Can you work these out from the model? Positions are in its coordinate system, mm. A direction names the side the tool comes from. Coordinates: 2 decimals unless noted, no trailing zeros. Order: outer loops, then holes, each group sorted by start corner. A loop starts at its lowest first (then second) coordinate and runs counter-clockwise, first axis right, second up. Notation, with made-up numbers: (-34.5, 41) -> (-25.5, 41) arc R15 cw to (-25.5, 53) -> close; hole circle Ø6 at (7, -5). An arc over 180 degrees is marked (long way). Write item = value, one per line.
```python
from build123d import *

# Parameters (mm, degrees)
SKETCH1_R           = 31.35
SKETCH1_R_2         = 16.65
BOSS_EXTRUDE1_DEPTH = 3
SKETCH2_R           = 4.85
BOSS_EXTRUDE2_DEPTH = 18
CIRPATTERN1_COUNT   = 6
CHAMFER1_SIZE       = 0.6


with BuildPart() as part:
    # Sketch1 → Boss-Extrude1 (new body)
    with BuildSketch(Plane.XY):
        Circle(SKETCH1_R)
        Circle(SKETCH1_R_2, mode=Mode.SUBTRACT)
    extrude(amount=-BOSS_EXTRUDE1_DEPTH)

    # Sketch2 → Boss-Extrude2 (add)
    with BuildSketch(Plane.XY):
        with Locations((24, 0)):
            Circle(SKETCH2_R)
    boss_extrude2 = extrude(amount=BOSS_EXTRUDE2_DEPTH)

    # CirPattern1: Boss-Extrude2 ×6 about axis
    cirpattern1_axis = Axis((0, 0, 0), (0, 0, 1))
    for i in range(1, CIRPATTERN1_COUNT):
        add(boss_extrude2.rotate(cirpattern1_axis, i * 360 / CIRPATTERN1_COUNT))

    # Chamfer1
    chamfer1_edges = [part.edges().sort_by_distance(p)[0] for p in [
        (19.15, 0, 18),
        (9.575, -16.584386482, 18),
        (-9.575, -16.584386482, 18),
        (-31.35, 0, 0),
        (-19.15, 0, 18),
        (-9.575, 16.584386482, 18),
        (9.575, 16.584386482, 18),
        (-31.35, 0, -3),
        (-16.65, 0, -3),
        (-16.65, 0, 0),
    ]]
    chamfer(chamfer1_edges, length=CHAMFER1_SIZE)


solid = part.part
```
Item 1: I want a section at B-B, the plane y = 0. Please give me the cut outline in (x, z), plus the area to 3 significant figures.
A:
outline = (-31.35, -2.4) -> (-30.75, -3) -> (-17.25, -3) -> (-16.65, -2.4) -> (-16.65, -0.6) -> (-17.25, 0) -> (-19.15, 0) -> (-19.15, 17.4) -> (-19.75, 18) -> (-28.25, 18) -> (-28.85, 17.4) -> (-28.85, 0) -> (-30.75, 0) -> (-31.35, -0.6) -> close; (16.65, -2.4) -> (17.25, -3) -> (30.75, -3) -> (31.35, -2.4) -> (31.35, -0.6) -> (30.75, 0) -> (28.85, 0) -> (28.85, 17.4) -> (28.25, 18) -> (19.75, 18) -> (19.15, 17.4) -> (19.15, 0) -> (17.25, 0) -> (16.65, -0.6) -> close
area = 435 mm2
Item 2: I want a section at C-C, the plane z = 12. Please give me the cut outline in (x, y) (3 decimals).
A:
outline = circle Ø9.7 at (-24, 0); circle Ø9.7 at (-12, -20.785); circle Ø9.7 at (-12, 20.785); circle Ø9.7 at (12, -20.785); circle Ø9.7 at (12, 20.785); circle Ø9.7 at (24, 0)
Item 3: If we mould it in two halves opening along Y, with no side actions, what happens to faces 3 (the cylindrical face through (-7.52, 18.93, 8.58)), 4 (the cylindrical face through (7.52, -18.93, 8.58)), 5 (the cylindrical face through (-19.155, -0.213, 8.578)), 6 (the flat face through (-12, 21, 18))? For each: pulls with the +Y half, pulls with the -Y half, needs draft (parallel to the pull), parting line crosses it, or undercut.
A:
face_3 = undercut
face_4 = undercut
face_5 = parting line crosses it
face_6 = needs draft
Item 4: I'm going to push flat-ended pins straight in: P1, Ø1, axis at x = 7.5, y = 16.5, coming from the +Z side; P2, Ø10, axis at x = 9, z = 2, coming from the +Y side; P3, Ø6, axis at x = 11, z = 13, coming from the -Y side; P4, Ø18.5, axis at x = 5.5, y = 4.5, coming from the +Z side. Where does each tip first touch, or does it pass through?
A:
P1 = 0
P2 = 30.99
P3 = -25.63
P4 = through
Item 5: I want a section at A-A, the plane x = 0. Please give me the cut outline in (y, z), plus the area to 3 significant figures.
A:
outline = (-31.35, -2.4) -> (-30.75, -3) -> (-17.25, -3) -> (-16.65, -2.4) -> (-16.65, -0.6) -> (-17.25, 0) -> (-30.75, 0) -> (-31.35, -0.6) -> close; (16.65, -2.4) -> (17.25, -3) -> (30.75, -3) -> (31.35, -2.4) -> (31.35, -0.6) -> (30.75, 0) -> (17.25, 0) -> (16.65, -0.6) -> close
area = 86.8 mm2
Item 6: If I drill on probe 1 along Y at (x, z) = (0, -1.9); probe 2 along Z at (x, y) = (23, 17.5); probe 3 along Y at (x, z) = (13.5, 16.25), over which ranges is the centre line in solid material (lowest first)?
A:
probe_1 = -31.35 to -16.65, 16.65 to 31.35
probe_2 = -3 to 0
probe_3 = -25.4 to -16.17, 16.17 to 25.4
Item 7: For faces 1 (the flat face through (24, 0, 18)), 2 (the cylindrical face through (13.05, 25.52, 8.58)), which set-ups out of +Z, -Z, +X, -X, +Y, -Y let a thin tool reach every point of the face, with its end or its side?
A:
face_1 = +Z, +X, -X, +Y, -Y
face_2 = +Z
